The drawing under review shows one solid part. Ordinate dimensions are in mm from its lowest x, y, z. Give positions to 0.01 mm unless a question says otherwise; leave off trailing zeros. Loops run counter-clockwise (first coordinate to the right, second up) from the corner with the lowest first, then second, coordinate; pieces in that order, holes last. Notation, with made-up numbers: M -38.5,49 L -3.5,49 A31 cw -3.5,83 Z; hole C 87,15 d2. An arc over 180 degrees is marked long. One line per item, written item: value. Start each with the question number.
Q1. We need section C-C on y = 7. Write out the cut boundary in (x, z).
Q2. Mouldability with a two-part tool opening along Z and no side actions: class the marked faces 1, 2 and 3 as released by +Z, released by -Z, zero draft, split by the parting line, or undercut.
Q3. To check wall thickness, follow line 1 along Z through (x, y) = (2.5, 4.75); line 2 along X through (y, z) = (6, 1.65). State the ranges of each line that lie inside material, in increasing order. Write a range as from..to.
Q4. We need section A-A on z = 2.5. Write out the cut boundary in (x, y), plus the area to 3 significant figures.
Q5. We need section B-B on x = 2.5. Write out the cut boundary in (y, z).
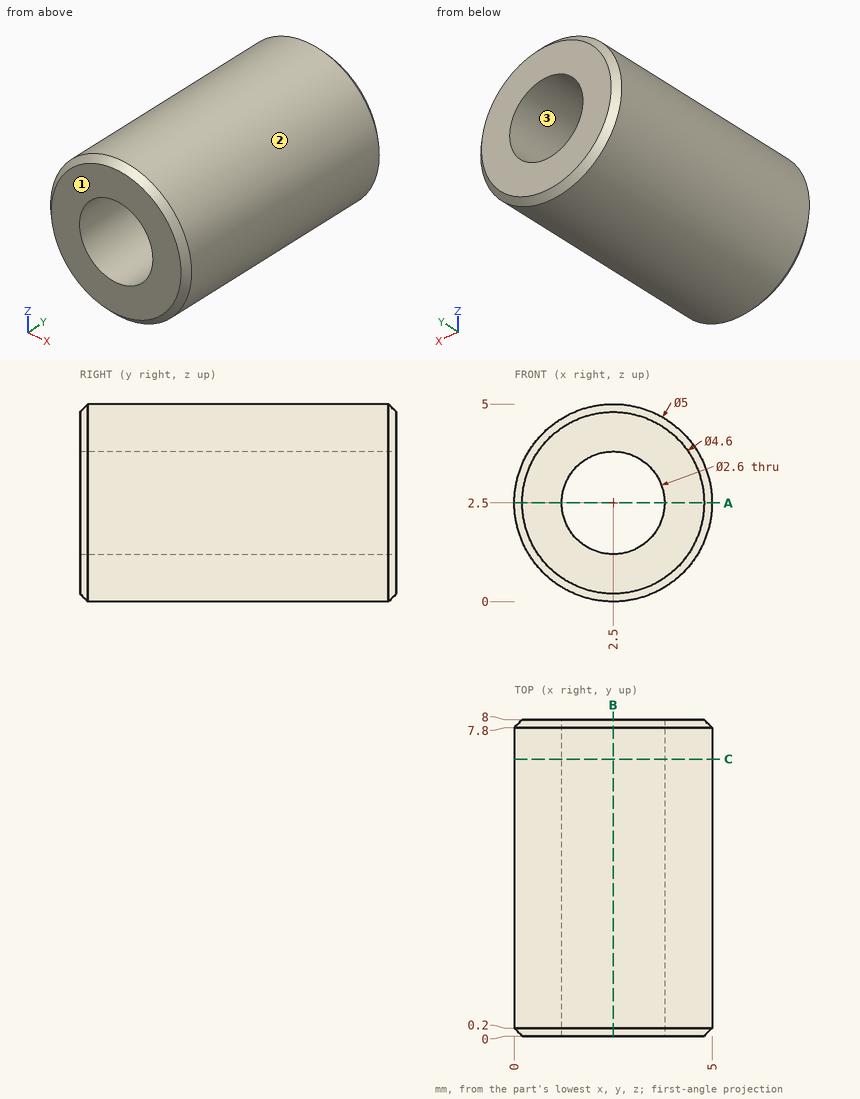
Solved:
1. outline: C 2.5,2.5 d5; hole C 2.5,2.5 d2.6
2. face 1: zero draft
2. face 2: split by the parting line
2. face 3: undercut
3. line 1: 0..1.2, 3.8..5
3. line 2: 0.15..1.52, 3.48..4.85
4. outline: M 0,0.2 L 0.2,0 L 1.2,0 L 1.2,8 L 0.2,8 L 0,7.8 Z; M 3.8,0 L 4.8,0 L 5,0.2 L 5,7.8 L 4.8,8 L 3.8,8 Z
4. area: 19.1 mm2
5. outline: M 0,0.2 L 0.2,0 L 7.8,0 L 8,0.2 L 8,1.2 L 0,1.2 Z; M 0,3.8 L 8,3.8 L 8,4.8 L 7.8,5 L 0.2,5 L 0,4.8 Z
